from build123d import *

# Parameters (mm, degrees)
BOSS_EXTRUDE1_DEPTH  = 20
SKETCH3_W            = 10
SKETCH3_H            = 40
BOSS_EXTRUDE2_DEPTH  = 60
SKETCH4_W            = 40
SKETCH4_H            = 40
CUT_EXTRUDE1_DEPTH   = 5
SKETCH5_R            = 15
BOSS_EXTRUDE3_DEPTH  = 5
SKETCH6_W            = 7.5
SKETCH6_H            = 5
BOSS_EXTRUDE4_DEPTH  = 20
SKETCH7_W            = 10
SKETCH7_H            = 5
BOSS_EXTRUDE5_DEPTH  = 5
SKETCH9_R            = 2.5
BOSS_EXTRUDE6_DEPTH  = 20
FILLET2_R            = 2.5
FILLET3_R            = 20
FILLET4_R            = 2.5
SKETCH10_W           = 30
SKETCH10_H           = 5
BOSS_EXTRUDE9_DEPTH  = 100
SKETCH12_W           = 7.5
SKETCH12_H           = 5
BOSS_EXTRUDE10_DEPTH = 20
SKETCH13_W           = 10
SKETCH13_H           = 5
BOSS_EXTRUDE11_DEPTH = 5
BOSS_EXTRUDE12_START = -15
SKETCH14_R           = 2.5
BOSS_EXTRUDE12_DEPTH = 20
SKETCH15_W           = 30
SKETCH15_H           = 5
BOSS_EXTRUDE13_DEPTH = 100
BOSS_EXTRUDE14_DEPTH = 20
BOSS_EXTRUDE15_START = -20
SKETCH17_W           = 10
SKETCH17_H           = 15
BOSS_EXTRUDE15_DEPTH = 30
CUT_EXTRUDE2_REACH   = 279.669
SKETCH18_W           = 10
SKETCH18_H           = 5
SKETCH19_R           = 2.5
CUT_EXTRUDE3_DEPTH   = 10
FILLET5_R            = 5
FILLET6_R            = 2.5


# Some blends are built 0.0001 mm under size
with BuildPart() as part:
    # Sketch1 → Boss-Extrude1 (new body)
    with BuildSketch(Plane(origin=(0, 0, 0), x_dir=(0, 0, -1), z_dir=(1, 0, 0))):
        with BuildLine():
            Line((-45, 0), (-50, 0))
            ThreePointArc((-50, 0), (0, 50), (50, 0))
            Line((50, 0), (45, 0))
            ThreePointArc((45, 0), (0, 45), (-45, 0))
        make_face()
    extrude(amount=BOSS_EXTRUDE1_DEPTH)

    # Sketch3 → Boss-Extrude2 (add)
    with BuildSketch(Plane(origin=(0, 0, 0), x_dir=(0, 0, -1), z_dir=(1, 0, 0))):
        with Locations((50, 0)):
            Rectangle(SKETCH3_W, SKETCH3_H)
    boss_extrude2 = extrude(amount=BOSS_EXTRUDE2_DEPTH)

    # Sketch4 → Cut-Extrude1 (cut)
    with BuildSketch(Plane.XY.offset(-45)):
        with Locations((40, 0)):
            Rectangle(SKETCH4_W, SKETCH4_H)
    cut_extrude1 = extrude(amount=-CUT_EXTRUDE1_DEPTH, mode=Mode.SUBTRACT)

    # Sketch5 → Boss-Extrude3 (add)
    with BuildSketch(Plane.XY.offset(-50)):
        with Locations(Location((40, 0, 0), (0, 0, 180))):
            Circle(SKETCH5_R)
    boss_extrude3 = extrude(amount=BOSS_EXTRUDE3_DEPTH)

    # Sketch6 → Boss-Extrude4 (add)
    with BuildSketch(Plane.ZY):
        with Locations((-3.75, 47.5)):
            Rectangle(SKETCH6_W, SKETCH6_H)
    boss_extrude4 = extrude(amount=BOSS_EXTRUDE4_DEPTH)

    # Sketch7 → Boss-Extrude5 (add)
    with BuildSketch(Plane(origin=(0, 0, -7.5), x_dir=(-1, 0, 0), z_dir=(0, 0, -1))):
        with Locations((10, 47.5)):
            Rectangle(SKETCH7_W, SKETCH7_H)
    boss_extrude5 = extrude(amount=BOSS_EXTRUDE5_DEPTH)

    # Sketch9 → Boss-Extrude6 (add)
    with BuildSketch(Plane(origin=(0, 0, 0), x_dir=(0, 0, -1), z_dir=(1, 0, 0))):
        with Locations((12.5, 47.5)):
            Circle(SKETCH9_R)
    boss_extrude6 = extrude(amount=-BOSS_EXTRUDE6_DEPTH)

    # Mirror1: Boss-Extrude2, Cut-Extrude1, Boss-Extrude3, Boss-Extrude4, Boss-Extrude5, Boss-Extrude6 across plane
    add(boss_extrude2.mirror(Plane.XY))
    add(cut_extrude1.mirror(Plane.XY), mode=Mode.SUBTRACT)
    add(boss_extrude3.mirror(Plane.XY))
    add(boss_extrude4.mirror(Plane.XY))
    add(boss_extrude5.mirror(Plane.XY))
    add(boss_extrude6.mirror(Plane.XY))

    # Fillet2
    fillet2_edges = [part.edges().sort_by_distance(p)[0] for p in [
        (20, 45, 0),
        (10, -20, 45),
        (20, -10, 45),
        (0, -20, -50),
        (10, -20, -45),
        (20, -10, -45),
        (0, -20, 50),
    ]]
    fillet(fillet2_edges, radius=FILLET2_R)

    # Fillet3
    fillet3_edges = [part.edges().sort_by_distance(p)[0] for p in [
        (60, -20, -52.5),
        (60, 20, -52.5),
        (60, -20, 52.5),
        (60, 20, 52.5),
    ]]
    fillet(fillet3_edges, radius=FILLET3_R - 0.0001)  # a hair under: the kernel refuses the full size

    # Fillet4
    fillet4_edges = [part.edges().sort_by_distance(p)[0] for p in [
        (30.00005, -20, 50),
        (30.00005, 20, -50),
        (54.142164913, 14.142164913, -50),
        (54.142164913, -14.142164913, -50),
        (30.00005, 20, 50),
        (54.142164913, 14.142164913, 50),
        (54.142164913, -14.142164913, 50),
        (30.00005, -20, -50),
    ]]
    fillet(fillet4_edges, radius=FILLET4_R)

    # Sketch10 → Boss-Extrude9 (add)
    with BuildSketch(Plane.ZY.offset(20)):
        with Locations((0, 47.5)):
            Rectangle(SKETCH10_W, SKETCH10_H)
    extrude(amount=BOSS_EXTRUDE9_DEPTH)

    # Sketch12 → Boss-Extrude10 (add)
    with BuildSketch(Plane.ZY.offset(120)):
        with Locations((-3.75, 47.5)):
            Rectangle(SKETCH12_W, SKETCH12_H)
    boss_extrude10 = extrude(amount=BOSS_EXTRUDE10_DEPTH)

    # Sketch13 → Boss-Extrude11 (add)
    with BuildSketch(Plane(origin=(0, 0, -7.5), x_dir=(-1, 0, 0), z_dir=(0, 0, -1))):
        with Locations((130, 47.5)):
            Rectangle(SKETCH13_W, SKETCH13_H)
    boss_extrude11 = extrude(amount=BOSS_EXTRUDE11_DEPTH)

    # Sketch14 → Boss-Extrude12 (add)
    with BuildSketch(Plane.ZY.offset(135).offset(BOSS_EXTRUDE12_START)):
        with Locations(Location((-12.5, 47.5, 0), (0, 0, 180))):
            Circle(SKETCH14_R)
    boss_extrude12 = extrude(amount=BOSS_EXTRUDE12_DEPTH)

    # Mirror2: Boss-Extrude10, Boss-Extrude11, Boss-Extrude12 across plane
    add(boss_extrude10.mirror(Plane(origin=(-140, 50, 0), x_dir=(1, 0, 0), z_dir=(0, 0, -1))))
    add(boss_extrude11.mirror(Plane(origin=(-140, 50, 0), x_dir=(1, 0, 0), z_dir=(0, 0, -1))))
    add(boss_extrude12.mirror(Plane(origin=(-140, 50, 0), x_dir=(1, 0, 0), z_dir=(0, 0, -1))))

    # Sketch15 → Boss-Extrude13 (add)
    with BuildSketch(Plane.ZY.offset(140)):
        with Locations((0, 47.5)):
            Rectangle(SKETCH15_W, SKETCH15_H)
    extrude(amount=BOSS_EXTRUDE13_DEPTH)

    # Sketch16 → Boss-Extrude14 (add)
    with BuildSketch(Plane.ZY.offset(240)):
        with BuildLine():
            Line((50, 0), (45, 0))
            ThreePointArc((45, 0), (0, 45), (-45, 0))
            Line((-45, 0), (-50, 0))
            ThreePointArc((-50, 0), (0, 50), (50, 0))
        make_face()
    extrude(amount=-BOSS_EXTRUDE14_DEPTH)

    # Sketch17 → Boss-Extrude15 (add)
    with BuildSketch(Plane.ZY.offset(240).offset(BOSS_EXTRUDE15_START)):
        with Locations((50, 7.5)):
            Rectangle(SKETCH17_W, SKETCH17_H)
    boss_extrude15 = extrude(amount=BOSS_EXTRUDE15_DEPTH)

    # Sketch18 → Cut-Extrude2 (cut, up to next)
    with BuildSketch(Plane.XY.offset(55), mode=Mode.PRIVATE) as cut_extrude2_sk1:
        with Locations((-245, 2.5)):
            Rectangle(SKETCH18_W, SKETCH18_H)
    cut_extrude2_tool1 = extrude(cut_extrude2_sk1.sketch, amount=-CUT_EXTRUDE2_REACH, mode=Mode.PRIVATE) & part.part
    cut_extrude2 = cut_extrude2_tool1.solids().sort_by_distance((-245, 2.5, 55))[0]
    add(cut_extrude2, mode=Mode.SUBTRACT)

    # Sketch19 → Cut-Extrude3 (cut)
    with BuildSketch(Plane.XZ.offset(-5)):
        with Locations(Location((-245, 50, 0), (0, 0, 270))):
            Circle(SKETCH19_R)
    cut_extrude3 = extrude(amount=-CUT_EXTRUDE3_DEPTH, mode=Mode.SUBTRACT)

    # Mirror3: Boss-Extrude15, Cut-Extrude2, Cut-Extrude3 across Top Plane
    add(boss_extrude15.mirror(Plane(origin=(0, 0, 0), x_dir=(1, 0, 0), z_dir=(0, 1, 0))))
    add(cut_extrude2.mirror(Plane(origin=(0, 0, 0), x_dir=(1, 0, 0), z_dir=(0, 1, 0))), mode=Mode.SUBTRACT)
    add(cut_extrude3.mirror(Plane(origin=(0, 0, 0), x_dir=(1, 0, 0), z_dir=(0, 1, 0))), mode=Mode.SUBTRACT)

    # Fillet5
    fillet5_edges = [part.edges().sort_by_distance(p)[0] for p in [
        (-250, -10, 45),
        (-250, -10, 55),
        (-250, 10, 55),
        (-250, 10, 45),
    ]]
    fillet(fillet5_edges, radius=FILLET5_R - 0.0001)  # a hair under: the kernel refuses the full size

    # Fillet6
    # the kernel refuses this fillet: 2.5 mm, written as the material it takes off along each edge
    with BuildSketch(Plane(origin=(-246.581228163, 0, -50), x_dir=(0, 0, 1), z_dir=(1, 0, 0))) as fillet6_piece_1:
        with BuildLine():
            CenterArc((2.565835097, -2.5), FILLET6_R, 90, 93.01696131)
            ThreePointArc((0.069300103, -2.631578947), (0.017328028, -1.316245633), (0, 0))
            Line((0, 0), (2.565835097, 0))
        make_face()
    extrude(amount=33.162456325, mode=Mode.SUBTRACT)
    with BuildSketch(Plane(origin=(-246.085412256, 0, -45), x_dir=(0, 0.9996534394348647, 0.026324912650289762), z_dir=(1, 0, 0))) as fillet6_piece_2:
        with BuildLine():
            CenterArc((2.43505442, -2.499133599), FILLET6_R, 91.508480655, 86.98303869)
            Line((-0.064079178, -2.433321317), (0, 0))
            ThreePointArc((0, 0), (1.184621069, -0.015595225), (2.369242139, 0))
        make_face()
    extrude(amount=32.170824513, mode=Mode.SUBTRACT)
    with BuildSketch(Plane(origin=(-213.75, -15, 45), x_dir=(0, 0, 1), z_dir=(-1, 0, 0)), Plane(origin=(-213.75, -15, 55), x_dir=(0, 1, 0), z_dir=(-1, 0, 0))) as fillet6_piece_3:
        with BuildLine():
            CenterArc((FILLET6_R, FILLET6_R), FILLET6_R, 180, 90)
            Line((0, FILLET6_R), (0, 0))
            Line((0, 0), (FILLET6_R, 0))
        make_face()
    extrude(amount=31.2501, mode=Mode.SUBTRACT)
    with BuildSketch(Plane(origin=(-245.0001, -15, 50.0001), x_dir=(0, 0, 1), z_dir=(1, 0, 0))) as fillet6_piece_4:
        with BuildLine():
            CenterArc((4.9999 - FILLET6_R, -FILLET6_R), FILLET6_R, 0, 90)
            Line((4.9999, -FILLET6_R), (4.9999, 0))
            Line((4.9999, 0), (4.9999 - FILLET6_R, 0))
        make_face()
    revolve(axis=Axis((-245.0001, -15, 50.0001), (0, -1, 0)), revolution_arc=90, mode=Mode.SUBTRACT)
    with BuildSketch(Plane(origin=(-245.0001, -15, 49.9999), x_dir=(0, 0, -1), z_dir=(1, 0, 0))) as fillet6_piece_5:
        with BuildLine():
            CenterArc((4.9999 - FILLET6_R, FILLET6_R), FILLET6_R, 270, 90)
            Line((4.9999, FILLET6_R), (4.9999, 0))
            Line((4.9999, 0), (4.9999 - FILLET6_R, 0))
        make_face()
    revolve(axis=Axis((-245.0001, -15, 49.9999), (0, 1, 0)), revolution_arc=90, mode=Mode.SUBTRACT)
    with BuildSketch(Plane(origin=(-250, -15, 50.0001), x_dir=(1, 0, 0), z_dir=(0, 0, -1))) as fillet6_piece_6:
        with BuildLine():
            CenterArc((FILLET6_R, -FILLET6_R), FILLET6_R, 90, 90)
            Line((0, -FILLET6_R), (0, 0))
            Line((0, 0), (FILLET6_R, 0))
        make_face()
    extrude(amount=0.0002, mode=Mode.SUBTRACT)


solid = part.part
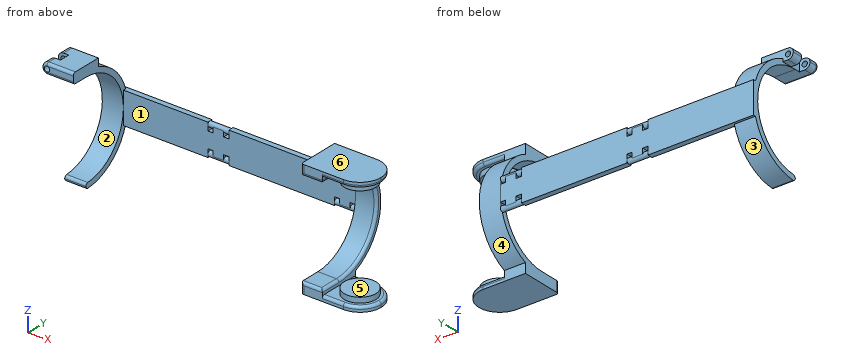
CAD build for the part. Positions are in the model's coordinates, mm. Face numbers are marked on the shaded views. A direction names the side the tool comes from. Give positions to 0.01 mm unless a question says otherwise; leave off trailing zeros. Write each loop counter-clockwise with the first axis right and the second up, starting at its lowest first coordinate (ties: lowest second). Pieces come first, ordered by that corner, then holes. Notation, with made-up numbers: (44.25, -11) -> (81.25, -11) arc R23 cw to (81.25, 28) -> close; hole circle Ø3 at (63.25, 43). An arc over 180 degrees is marked (long way). Return JSON: item names as keys, results as strings.
Item 1: Drop flat-ended pins along their axis: pin 1 (0.8 mm diameter, centred on y = 49, z = -14, fed in from -X); pin 2 (8 mm diameter, centred on x = -244, z = 49.5, fed in from -Y); pin 3 (2.5 mm diameter, centred on y = 47, z = 9.5, fed in from +X). Give the stop position or say it passes through.
Answer below:
{"pin 1": "stops at x = -240", "pin 2": "stops at y = -15", "pin 3": "stops at x = 20"}
Item 2: Band-saw the part on B-B (y = 32.5). Give the number of separate pieces and of enclosed holes in the cut face, then the cut area to 3 significant figures.
Answer below:
{"separate pieces": "4", "enclosed holes": "0", "area": "546 mm2"}
Item 3: Band-saw the part on C-C (x = -115). List the corners of the cut face in (y, z).
Answer below:
{"outline": "(45, -15) -> (50, -15) -> (50, 15) -> (45, 15) -> close"}
Item 4: Two-plate mould, pull along Z, no slides. Class the marked faces 4, 5 and 6: +Z half, -Z half, draft (parallel to the pull), parting line (faces both ways), or undercut.
Answer below:
{"face 4": "parting line", "face 5": "undercut", "face 6": "+Z half"}
Item 5: Drill centre lines: probe 1 along Z at (x, y) = (-245, 11.75); probe 2 along Z at (x, y) = (0.5, 19); probe 3 along Y at (x, z) = (-29.5, -1). Where is each one in solid material? Low to high.
Answer below:
{"probe 1": "z = 45 to 47.5, 52.5 to 55", "probe 2": "z = -55 to -40.79, 40.79 to 55", "probe 3": "y = 45 to 50"}
Item 6: Tool access for the marked faces 1, 2 and 3: list every direction of +Z, -Z, +X, -X, +Y, -Y with a clear straight run to the whole face (end or side of a thin tool).
Answer below:
{"face 1": "+Z, -Z, -Y", "face 2": "+X, -X, -Y", "face 3": "-Z, -X, +Y"}
Item 7: Band-saw the part on A-A (x = -223.5). List the corners of the cut face in (y, z), then the cut area to 4 significant figures.
Answer below:
{"outline": "(-15, 47.5) arc R2.5 ccw to (-12.5, 45) -> (0, 45) arc R45 cw to (2.37, -44.94) arc R2.5 ccw to (2.63, -49.93) arc R50 ccw to (47.7, -15) -> (50, -15) -> (50, 15) -> (47.7, 15) arc R50 ccw to (15, 47.7) -> (15, 55) -> (-12.5, 55) arc R2.5 ccw to (-15, 52.5) -> close", "area": "1,000 mm2"}
